Source: CAD feature listing. Evaluate the final solid. Frame: model axes, mm. Face numbers are marked on the shaded views. A direction names the side the tool comes from. Round coordinates to 2 decimals unless told otherwise and drop trailing zeros. Order: outer loops, then holes, each group sorted by start corner. A loop starts at its lowest first (then second) coordinate and runs counter-clockwise, first axis right, second up. Notation, with made-up numbers: (7.25, 47) - (25.25, 47) arc R16 cw to (25.25, 62) - close; hole circle Ø1 at (64, 76). An arc over 180 degrees is marked (long way). Use one line per item in the form item = value. Start each with the question number.
Q1. Set-up query: the marked faces 1 and 2. Return all of +Z, -Z, +X, -X, +Y, -Y with unobstructed straight access to the full face (end or side cutting, diameter ignored); none if empty.
Q2. Pin query (flat end, axial travel): pin 1 Ø4 at (x, y) = (13, 6.5) entering from +Z; pin 2 Ø1.2 at (x, y) = (2, -2) entering from -Z; pin 3 Ø1.2 at (x, y) = (2, -1.5) entering from +Z. Return the tip coordinate at first contact, or that it passes through.
Q3. Cut plane D-D, the plane x = 13.5. Return the cut outline in (y, z).
Q4. Cut plane A-A, the plane y = -2. Return the cut outline in (x, z), and give its area (3 significant figures).
Q5. Cut plane C-C, the plane z = 0. Return the cut outline in (x, y).
Q6. Ray query, line 1 (Y direction, x = 16, z = 0); line 2 (Z direction, x = 19, y = 4.25); line 3 (Z direction, x = 2, y = -0.5). Return the intervals inside material, ascending. Write a range as [from, to].
Q7. Cut plane B-B, the plane x = -4.95. Return the cut outline in (y, z), and give its area (3 significant figures).
Q8. Draft query along Z for the marked faces 3, 4 and 5. Return one class per face: released by +Z, released by -Z, zero draft, split by the parting line, or undercut.
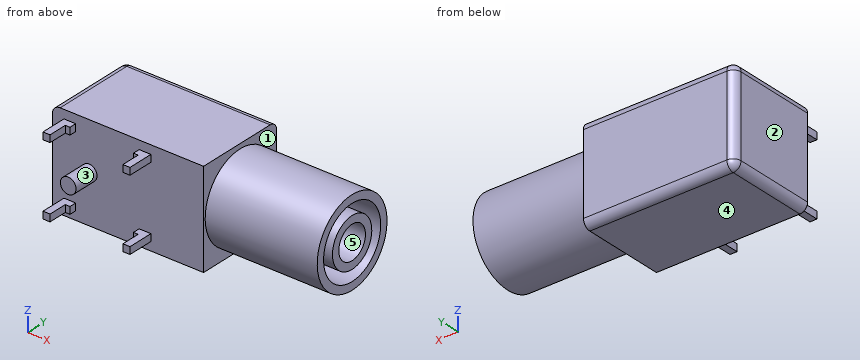
from build123d import *

# Parameters (mm, degrees)
SKETCH_1_W               = 19.3
SKETCH_1_H               = 12.2
EXTRUDE_1_DEPTH          = 11.5
FILLET_4_R               = 1
SKETCH_2_R               = 5.5
EXTRUDE_2_DEPTH          = 14.3
SKETCH_3_R               = 4.5
CUT_EXTRUDE_1_DEPTH      = 14.3
SKETCH_4_R               = 3.1
SKETCH_4_R_2             = 2.1
EXTRUDE_3_DEPTH          = 14.3
SKETCH_5_W               = 1.5
SKETCH_5_H               = 0.9
EXTRUDE_4_DEPTH          = 0.9
SKETCH_6_W               = 0.9
SKETCH_6_H               = 0.9
EXTRUDE_5_DEPTH          = 2.4
PATTERN_LINEAR_1_COUNT   = 2
PATTERN_LINEAR_1_PITCH   = 9.1
MIRROR_1_COPY_1_SKETCH_W = 1.5
MIRROR_1_COPY_1_SKETCH_H = 0.9
MIRROR_1_COPY_1_DEPTH    = 0.9
MIRROR_1_COPY_2_SKETCH_W = 0.9
MIRROR_1_COPY_2_SKETCH_H = 0.9
MIRROR_1_COPY_2_DEPTH    = 2.4
SKETCH_7_R               = 1
EXTRUDE_6_DEPTH          = 3.3


with BuildPart() as part:
    # Эскиз1 → Бобышка-Вытянуть1 (new body)
    with BuildSketch(Plane(origin=(0, 0, 0), x_dir=(1, 0, 0), z_dir=(0, 1, 0))):
        Rectangle(SKETCH_1_W, SKETCH_1_H)
    extrude(amount=EXTRUDE_1_DEPTH)

    # Скругление4
    fillet_4_edges = [part.edges().sort_by_distance(p)[0] for p in [
        (-9.65, 11.5, 0),
        (0, 11.5, 6.1),
        (-9.65, 5.75, 6.1),
        (-9.65, 5.75, -6.1),
        (0, 11.5, -6.1),
    ]]
    fillet(fillet_4_edges, radius=FILLET_4_R)

    # Эскиз2 → Бобышка-Вытянуть2 (add)
    with BuildSketch(Plane(origin=(9.65, 0, 0), x_dir=(0, 0, -1), z_dir=(1, 0, 0))):
        with Locations((0, 5.75)):
            Circle(SKETCH_2_R)
    extrude(amount=EXTRUDE_2_DEPTH)

    # Эскиз3 → Вырез-Вытянуть1 (cut)
    with BuildSketch(Plane(origin=(23.95, 0, 0), x_dir=(0, 0, -1), z_dir=(1, 0, 0))):
        with Locations((0, 5.75)):
            Circle(SKETCH_3_R)
    extrude(amount=-CUT_EXTRUDE_1_DEPTH, mode=Mode.SUBTRACT)

    # Эскиз4 → Бобышка-Вытянуть3 (add)
    with BuildSketch(Plane(origin=(9.65, 0, 0), x_dir=(0, 0, -1), z_dir=(1, 0, 0))):
        with Locations((0, 5.75)):
            Circle(SKETCH_4_R)
        with Locations((0, 5.75)):
            Circle(SKETCH_4_R_2, mode=Mode.SUBTRACT)
    extrude(amount=EXTRUDE_3_DEPTH)

    # Эскиз5 → Бобышка-Вытянуть4 (add)
    with BuildSketch(Plane.XZ):
        with Locations((-7.42, 4.55)):
            Rectangle(SKETCH_5_W, SKETCH_5_H)
    extrude_4 = extrude(amount=EXTRUDE_4_DEPTH)

    # Эскиз6 → Бобышка-Вытянуть5 (add)
    with BuildSketch(Plane.XZ.offset(0.9)):
        with Locations((-7.72, 4.55)):
            Rectangle(SKETCH_6_W, SKETCH_6_H)
    extrude_5 = extrude(amount=EXTRUDE_5_DEPTH)

    # Линейный массив1: Бобышка-Вытянуть4, Бобышка-Вытянуть5 ×2
    with Locations(*[(0, 0, -i * PATTERN_LINEAR_1_PITCH) for i in range(1, PATTERN_LINEAR_1_COUNT)]):
        add(extrude_4)
        add(extrude_5)

    # Зеркальное отражение1: Бобышка-Вытянуть4, Бобышка-Вытянуть5 across plane
    add(extrude_4.mirror(Plane(origin=(-2.62, 0, 0), x_dir=(0, 0, 1), z_dir=(1, 0, 0))))
    add(extrude_5.mirror(Plane(origin=(-2.62, 0, 0), x_dir=(0, 0, 1), z_dir=(1, 0, 0))))

    # Зеркальное отражение1 copy 1 sketch → Зеркальное отражение1 copy 1 (add)
    with BuildSketch(Plane(origin=(-5.24, 0, -9.1), x_dir=(-1, 0, 0), z_dir=(0, -1, 0))):
        with Locations((-7.42, -4.55)):
            Rectangle(MIRROR_1_COPY_1_SKETCH_W, MIRROR_1_COPY_1_SKETCH_H)
    extrude(amount=MIRROR_1_COPY_1_DEPTH)

    # Зеркальное отражение1 copy 2 sketch → Зеркальное отражение1 copy 2 (add)
    with BuildSketch(Plane(origin=(-5.24, -0.9, -9.1), x_dir=(-1, 0, 0), z_dir=(0, -1, 0))):
        with Locations((-7.72, -4.55)):
            Rectangle(MIRROR_1_COPY_2_SKETCH_W, MIRROR_1_COPY_2_SKETCH_H)
    extrude(amount=MIRROR_1_COPY_2_DEPTH)

    # Эскиз7 → Бобышка-Вытянуть6 (add)
    with BuildSketch(Plane.XZ):
        with Locations(Location((-4.95, 0, 0), (0, 0, 90))):
            Circle(SKETCH_7_R)
    extrude(amount=EXTRUDE_6_DEPTH)


solid = part.part
Completed:
q1.face_1 = +X
q1.face_2 = +Z, -Z, -X, +Y, -Y
q2.pin_1 = 5.5
q2.pin_2 = -5
q2.pin_3 = 5
q3.outline = circle Ø11 at (5.75, 0); circle Ø6.2 at (5.75, 0); hole circle Ø9 at (5.75, 0); hole circle Ø4.2 at (5.75, 0)
q4.outline = (-8.17, -5) - (-7.27, -5) - (-7.27, -4.1) - (-8.17, -4.1) - close; (-8.17, 4.1) - (-7.27, 4.1) - (-7.27, 5) - (-8.17, 5) - close; circle Ø2 at (-4.95, 0); (2.03, -5) - (2.93, -5) - (2.93, -4.1) - (2.03, -4.1) - close; (2.03, 4.1) - (2.93, 4.1) - (2.93, 5) - (2.03, 5) - close
q4.area = 6.38 mm2
q5.outline = (-9.65, 0) - (-5.95, 0) - (-5.95, -3.3) - (-3.95, -3.3) - (-3.95, 0) - (9.65, 0) - (9.65, 0.25) - (23.95, 0.25) - (23.95, 1.25) - (9.65, 1.25) - (9.65, 2.65) - (23.95, 2.65) - (23.95, 3.65) - (9.65, 3.65) - (9.65, 7.85) - (23.95, 7.85) - (23.95, 8.85) - (9.65, 8.85) - (9.65, 10.25) - (23.95, 10.25) - (23.95, 11.25) - (9.65, 11.25) - (9.65, 11.5) - (-8.65, 11.5) arc R1 ccw to (-9.65, 10.5) - close
q6.line_1 = [0.25, 1.25], [2.65, 3.65], [7.85, 8.85], [10.25, 11.25]
q6.line_2 = [-5.29, -4.24], [-2.71, -1.47], [1.47, 2.71], [4.24, 5.29]
q6.line_3 = [-5, -4.1], [4.1, 5]
q7.outline = (-3.3, -1) - (0, -1) - (0, -6.1) - (10.5, -6.1) arc R1 ccw to (11.5, -5.1) - (11.5, 5.1) arc R1 ccw to (10.5, 6.1) - (0, 6.1) - (0, 1) - (-3.3, 1) - close
q7.area = 146 mm2
q8.face_3 = split by the parting line
q8.face_4 = released by -Z
q8.face_5 = undercut
